Geometry check sheet. Reference: the model listing, model coordinates, mm. A direction names the side the tool comes from. Coordinates: 2 decimals unless noted, no trailing zeros. Order: outer loops, then holes, each group sorted by start corner. A loop starts at its lowest first (then second) coordinate and runs counter-clockwise, first axis right, second up. Notation, with made-up numbers: M 55.5,-40 L 72.5,-40 A20 ccw 72.5,-25 Z; hole C 89,-14.75 d5. An arc over 180 degrees is marked long. Use CSV: the item, a comma, the result in double quotes. Start each with the question number.
```python
from build123d import *

# Parameters (mm, degrees)
SKETCH031_W  = 7
SKETCH031_H  = 43
SKETCH029_W  = 47
SKETCH029_H  = 43
PAD006_DEPTH = 31
PAD007_DEPTH = 3
PAD013_DEPTH = 3


with BuildPart() as part:
    # Sketch031 → AdditiveLoft001 section 0
    with BuildSketch(Plane(origin=(0, 0, -31.2), x_dir=(1, 0, 0), z_dir=(0, 0, -1))):
        with Locations((-41.5, 0)):
            Rectangle(SKETCH031_W, SKETCH031_H)
    # Sketch029 → AdditiveLoft001 section 1
    with BuildSketch(Plane.XY.offset(-0.2)):
        with Locations((-41.5, 0)):
            Rectangle(SKETCH029_W, SKETCH029_H)
    loft()

    # Sketch027 → Pad006 (new body)
    with BuildSketch(Plane(origin=(0, 0, -31.2), x_dir=(1, 0, 0), z_dir=(0, 0, -1))):
        Polygon((-18, 16.5), (-38, 16.5), (-38, -16.5), (-19.5, -16.5), (-19.5, -20.2), (-26.5, -20.2), (-26.5, -21.5), (-65, -21.5), (-65, -16.5), (-45, -16.5), (-45, 16.5), (-63.4, 16.5), (-63.4, 20.2), (-56.4, 20.2), (-56.4, 21.5), (-18, 21.5), align=None)
    extrude(amount=-PAD006_DEPTH)

    # Sketch035 → Pad007 (join)
    with BuildSketch(Plane.XY.offset(-0.2)):
        Polygon((-24, 21.5), (-24, 20.3), (-19.2, 20.3), (-19.2, 14.5), (-18, 14.5), (-18, 21.5), align=None)
    extrude(amount=PAD007_DEPTH)

    # Sketch032 (on Face11 of Pad007) → Pad013 (join)
    with BuildSketch(Plane.XY.offset(-0.2)):
        Polygon((-65, -14.5), (-65, -21.5), (-59, -21.5), (-59, -20.3), (-63.8, -20.3), (-63.8, -14.5), align=None)
    extrude(amount=PAD013_DEPTH)


solid = part.part
```
1) Material ranges on line 1 along Y through (x, z) = (-55, -20); line 2 along Y through (x, z) = (-22.5, -22.5); line 3 along Z through (x, y) = (-41.5, 9), recorded low to high.
2) Set-up check for faces 1 (the face through (-19.5, 18, -17)), 2 (the face through (-59, -21, 1)), 3 (the face through (-58, -16.5, -23)): record each of +Z, -Z, +X, -X, +Y, -Y from which the full face is reachable in a straight line by a thin tool's end or side.
3) Section check B-B on x = -50. Record the boundary of the cut face in (y, z), then the cut area to 3 significant figures.
4) Draft check along Y on faces 4 (the face through (-63.8, -17, 1)), 5 (the face through (-27.86, 2.77, -15.48)), 6 (the face through (-46, 21.5, -14)). Enter one of: +Y half, -Y half, draft (parallel to the pull), parting line (faces both ways), or undercut.
5) Section check C-C on z = -25. Record the boundary of the cut face in (x, y), then the cut area to 3 significant figures.
6) Gauge pin test, flat ends, axial feed: P1, Ø10, axis at x = -25.5, y = -3, coming from the +Z side; P2, Ø1, axis at x = -34.5, y = -9, coming from the -Z side; P3, Ø2.5, axis at x = -61.5, z = 1.5, coming from the +Y side. Record the tip position at first contact, or that the pin passes through.
7) Section check D-D on y = 4.5. Record the boundary of the cut face in (x, z), then the cut area to 3 significant figures.
8) Section check A-A on z = 0.5. Record the boundary of the cut face in (x, y).
Results are:
1,line 1,"y = -21.5 to -16.5, 16.5 to 21.5"
1,line 2,"y = -21.5 to -16.5, 16.5 to 20.2"
1,line 3,"z = -31.2 to -0.2"
2,face 1,"-Z, +X, +Y"
2,face 2,"+Z, +X, +Y, -Y"
2,face 3,"-Z, -X"
3,outline,"M -21.5,-31.2 L -16.5,-31.2 L -16.5,-23.45 L 16.5,-23.45 L 16.5,-31.2 L 21.5,-31.2 L 21.5,-0.2 L -21.5,-0.2 Z"
3,area,"1,080 mm²"
4,face 4,"draft"
4,face 5,"undercut"
4,face 6,"+Y half"
5,outline,"M -65,16.5 L -49,16.5 L -49,-16.5 L -63.4,-16.5 L -63.4,-20.2 L -56.4,-20.2 L -56.4,-21.5 L -18,-21.5 L -18,-16.5 L -34,-16.5 L -34,16.5 L -19.5,16.5 L -19.5,20.2 L -26.5,20.2 L -26.5,21.5 L -65,21.5 Z"
5,area,"931 mm²"
6,P1,"stops at z = -0.2"
6,P2,"stops at z = -26.55"
6,P3,"stops at y = -20.3"
7,outline,"M -65,-0.2 L -45,-31.2 L -38,-31.2 L -18,-0.2 Z"
7,area,"837 mm²"
8,outline,"M -65,-21.5 L -59,-21.5 L -59,-20.3 L -63.8,-20.3 L -63.8,-14.5 L -65,-14.5 Z; M -24,20.3 L -19.2,20.3 L -19.2,14.5 L -18,14.5 L -18,21.5 L -24,21.5 Z"
